from build123d import *

# Parameters (mm, degrees)
SKETCH1_W           = 53
SKETCH1_H           = 29
BOSS_EXTRUDE1_DEPTH = 1
SKETCH2_W           = 52
SKETCH2_H           = 28
BOSS_EXTRUDE2_DEPTH = 1
SHELL1_START        = -1
SHELL1_OUTLINE_W    = 50
SHELL1_OUTLINE_H    = 26
SHELL1_DEPTH        = 1


# Read off the part's stored shape, not the designer's step: Shell1
with BuildPart() as part:
    # Sketch1 → Boss-Extrude1 (new body)
    with BuildSketch(Plane.XY):
        Rectangle(SKETCH1_W, SKETCH1_H)
    extrude(amount=BOSS_EXTRUDE1_DEPTH)

    # Sketch2 → Boss-Extrude2 (add)
    with BuildSketch(Plane(origin=(0, 0, 0), x_dir=(-1, 0, 0), z_dir=(0, 0, -1))):
        Rectangle(SKETCH2_W, SKETCH2_H)
    extrude(amount=BOSS_EXTRUDE2_DEPTH)

    # Shell1 outline → Shell1 (cut)
    with BuildSketch(Plane.XY.offset(SHELL1_START)):
        Rectangle(SHELL1_OUTLINE_W, SHELL1_OUTLINE_H)
    extrude(amount=SHELL1_DEPTH, mode=Mode.SUBTRACT)


solid = part.part
Check sheet for the modelled part. Datum: model origin and axes. Units: mm. A direction names the side the tool comes from. Give positions to 0.01 mm unless a question says otherwise; leave off trailing zeros. Write each loop counter-clockwise with the first axis right and the second up, starting at its lowest first coordinate (ties: lowest second). Pieces come first, ordered by that corner, then holes. Notation, with made-up numbers: (-33, 89) -> (-27, 89) arc R17 ccw to (-27, 115) -> close; hole circle Ø1 at (54, 59). An arc over 180 degrees is marked (long way). One line per item, written item: value. Start each with the question number.
Item 1: Section check B-B on z = -0.55. Record the cut outline in (x, y), then the cut area to 3 significant figures.
Item 2: Tool access check on faces 1 (the flat face through (-0.3, -13, -0.5)), 2 (the flat face through (26, -0.2, -0.5)), 3 (the flat face through (-26, -0.2, -0.5)). Record the directions out of +Z, -Z, +X, -X, +Y, -Y that give a thin tool (end or side, any length) a straight path to the whole face; none if there is none.
Item 3: Material ranges on probe 1 along X at (y, z) = (-8.75, -0.15); probe 2 along Y at (x, z) = (16.5, -0.2); probe 3 along Z at (x, y) = (-2, -9), recorded low to high. Write a range as from..to.
Item 4: Draft check along Y on faces 4 (the flat face through (7.8, 13.5, -1)), 5 (the flat face through (0.4, -14, -0.5)), 6 (the flat face through (-25, -0.2, -0.5)). Enter one of: +Y half, -Y half, draft (parallel to the pull), parting line (faces both ways), or undercut.
Item 5: Section check C-C on x = -20.5. Record the cut outline in (y, z), then the cut area to 3 significant figures.
Item 6: Gauge pin test, flat ends, axial feed: pin 1 (4 mm diameter, centred on x = -0.5, y = -3.5, fed in from -Z); pin 2 (0.8 mm diameter, centred on y = -0.5, z = -0.5, fed in from +X); pin 3 (0.5 mm diameter, centred on x = 3, z = -0.5, fed in from +Y). Record the tip position at first contact, or that the pin passes through.
Item 7: Section check A-A on y = 9.25. Record the cut outline in (x, z), then the cut area to 3 significant figures.
Results list:
1. outline: (-26, -14) -> (26, -14) -> (26, 14) -> (-26, 14) -> close; hole (-25, -13) -> (25, -13) -> (25, 13) -> (-25, 13) -> close
1. area: 156 mm²
2. face 1: -Z
2. face 2: -Z, +X, +Y, -Y
2. face 3: -Z, -X, +Y, -Y
3. probe 1: -26..-25, 25..26
3. probe 2: -14..-13, 13..14
3. probe 3: 0..1
4. face 4: draft
4. face 5: -Y half
4. face 6: undercut
5. outline: (-14.5, 0) -> (-14, 0) -> (-14, -1) -> (-13, -1) -> (-13, 0) -> (13, 0) -> (13, -1) -> (14, -1) -> (14, 0) -> (14.5, 0) -> (14.5, 1) -> (-14.5, 1) -> close
5. area: 31.0 mm²
6. pin 1: z = 0
6. pin 2: x = 26
6. pin 3: y = 14
7. outline: (-26.5, 0) -> (-26, 0) -> (-26, -1) -> (-25, -1) -> (-25, 0) -> (25, 0) -> (25, -1) -> (26, -1) -> (26, 0) -> (26.5, 0) -> (26.5, 1) -> (-26.5, 1) -> close
7. area: 55.0 mm²
